Can you work these out from the model? Positions are in its coordinate system, mm. A direction names the side the tool comes from. Coordinates: 2 decimals unless noted, no trailing zeros. Order: outer loops, then holes, each group sorted by start corner. A loop starts at its lowest first (then second) coordinate and runs counter-clockwise, first axis right, second up. Notation, with made-up numbers: (0, -33) -> (58, -33) arc R16 cw to (58, -27) -> close; hole circle Ø2 at (-40, 73.25). An arc over 180 degrees is marked (long way). Write item = value, one per line. Start each with the question number.
from build123d import *

# Parameters (mm, degrees)
GRIPPER_ATTACHMENT_BASE_SKETCH_W   = 12
GRIPPER_ATTACHMENT_BASE_SKETCH_H   = 15
GRIPPER_ATTACHMENT_BASE_DEPTH      = 35.0588586
THICKENER_BASE_DEPTH               = 6
THICKNESS_CUTOFF_SKETCH_W          = 51.475312709
THICKNESS_CUTOFF_SKETCH_H          = 66.937611181
THICKNESS_CUTOFF_DEPTH             = 63.622352222
EXCESS_MATERIAL_CUTOFF_DEPTH       = 530.479784495
EXCESS_MATERIAL_CUTOFF_DEPTH_BACK  = 530.479784495
FINGER_CAVITY_CUTOUT_SKETCH_W      = 6.5
FINGER_CAVITY_CUTOUT_SKETCH_H      = 22
FINGER_CAVITY_CUTOUT_DEPTH         = 15
SCREW_THROUGH_HOLES_SKETCH_R       = 2.25
SCREW_THROUGH_HOLES_DEPTH          = 63.800756824
SOCKET_RECESSES_SKETCH_R           = 3.75
SOCKET_RECESSES_DEPTH              = 2.3625
SHAPING_TO_ELECTRONICS_PLATE_DEPTH = 35.058859


with BuildPart() as part:
    # Gripper Attachment Base Sketch → Gripper Attachment Base (new body)
    with BuildSketch(Plane.XY):
        Rectangle(GRIPPER_ATTACHMENT_BASE_SKETCH_W, GRIPPER_ATTACHMENT_BASE_SKETCH_H)
    extrude(amount=GRIPPER_ATTACHMENT_BASE_DEPTH)

    # Thickener Base Sketch → Thickener Base (add)
    with BuildSketch(Plane(origin=(6, 0, 0), x_dir=(0, 0, -1), z_dir=(1, 0, 0))):
        with BuildLine():
            Line((0, 7.5), (-35.0588586, 7.5))
            Line((-35.0588586, 7.5), (-35.0588586, -48.8959251))
            ThreePointArc((-35.0588586, -48.8959251), (-17.5294293, -38.525001297), (0, -48.8959251))
            Line((0, -48.8959251), (0, 7.5))
        make_face()
    extrude(amount=THICKENER_BASE_DEPTH)

    # Thickness Cutoff Sketch → Thickness Cutoff (cut, through all)
    with BuildSketch(Plane(origin=(12.174072963, -0.29408868, 0), x_dir=(0, 0, -1), z_dir=(0.9997083481115524, -0.02414992165766464, 0))):
        with Locations((-17.603923241, -21.483184787)):
            Rectangle(THICKNESS_CUTOFF_SKETCH_W, THICKNESS_CUTOFF_SKETCH_H)
    extrude(amount=THICKNESS_CUTOFF_DEPTH, mode=Mode.SUBTRACT)

    # Excess Material Cutoff Sketch → Excess Material Cutoff (cut, two sides: drawn at the far end of the back side and taken through both)
    with BuildSketch(Plane(origin=(0, -520.681520523, 0), x_dir=(0, 0, 1), z_dir=(1, 0, 0)).offset(-EXCESS_MATERIAL_CUTOFF_DEPTH_BACK)):
        Polygon((7.0294293, -528.181520523), (0, -528.181520523), (0, -513.181520523), (7.0294293, -524.181520523), align=None)
        Polygon((28.0294293, -528.181520523), (35.0588586, -528.181520523), (35.0588586, -513.181520523), (28.0294293, -524.181520523), align=None)
    extrude(amount=EXCESS_MATERIAL_CUTOFF_DEPTH + EXCESS_MATERIAL_CUTOFF_DEPTH_BACK, mode=Mode.SUBTRACT)

    # Finger Cavity Cutout Sketch → Finger Cavity Cutout (cut)
    with BuildSketch(Plane(origin=(0, 7.5, 0), x_dir=(1, 0, 0), z_dir=(0, 1, 0))):
        with Locations((1.6125, -17.5294293)):
            Rectangle(FINGER_CAVITY_CUTOUT_SKETCH_W, FINGER_CAVITY_CUTOUT_SKETCH_H)
    extrude(amount=-FINGER_CAVITY_CUTOUT_DEPTH, mode=Mode.SUBTRACT)

    # Screw Through-Holes Sketch → Screw Through-Holes (cut, through all)
    with BuildSketch(Plane.ZY.offset(6)):
        with Locations(Location((11.5294293, -0.5, 0), (0, 0, 270))):
            Circle(SCREW_THROUGH_HOLES_SKETCH_R)
        with Locations(Location((23.5294293, -0.5, 0), (0, 0, 270))):
            Circle(SCREW_THROUGH_HOLES_SKETCH_R)
    extrude(amount=-SCREW_THROUGH_HOLES_DEPTH, mode=Mode.SUBTRACT)

    # Socket Recesses Sketch → Socket Recesses (cut)
    with BuildSketch(Plane.ZY.offset(6)):
        with Locations(Location((11.5294293, -0.5, 0), (0, 0, 270))):
            Circle(SOCKET_RECESSES_SKETCH_R)
        with Locations(Location((23.5294293, -0.5, 0), (0, 0, 270))):
            Circle(SOCKET_RECESSES_SKETCH_R)
    extrude(amount=-SOCKET_RECESSES_DEPTH, mode=Mode.SUBTRACT)

    # Shaping to Electronics Plate Sketch → Shaping to Electronics Plate (add, through all)
    with BuildSketch(Plane.XY):
        Polygon((-6, -7.5), (-3, -11.2), (-3, -7.5), align=None)
    extrude(amount=SHAPING_TO_ELECTRONICS_PLATE_DEPTH)


solid = part.part
(1) Imagine slicing it at D-D (z = 32.5). Write out the boundary of the cut face in (x, y).
(2) Thinking about a two-plate mould opening in Z: for faces 4 (the face through (-3.638, 0, 9)), 5 (the face through (2.874, -2.077, 3.466)), 6 (the face through (-4, -9, 35.059)), which applies, +Z half, -Z half, draft (parallel to the pull), parting line (faces both ways), or undercut?
(3) Imagine slicing it at C-C (z = 22.5). Write out the boundary of the cut face in (x, y), plus the area to 3 significant figures.
(4) Imagine slicing it at A-A (x = 2). Write out the boundary of the cut face in (y, z), plus the area to 3 significant figures.
(5) If I drill on L1, parallel to Z at x = -2.4, y = -0.5; L2, parallel to X at y = -6, z = 14.5; L3, parallel to Z at x = -5, y = -3, over which ranges is the centre line in solid material (lowest first)? Write a range as from..to.
(6) For faces 1 (the face through (8, 5, 28.029)), 2 (the face through (-3.638, 0, 21)), 3 (the face through (-1.638, 0, 18)), which set-ups out of +Z, -Z, +X, -X, +Y, -Y let a thin tool reach every point of the face, with its end or its side?
(7) For P1, Ø17.5, axis at y = -20.5, z = 20, coming from the -X side; P2, Ø10, axis at x = 4, z = 18.5, coming from the -Y side; P3, Ø7, axis at x = 2, y = -1.5, coming from the -Z side, each with a flat end and sliding along its axis, tell me the tip position at first contact or that it passes through.
(8) Imagine slicing it at B-B (y = -0.5). Count the separate pieces of the cut face and the enclosed holes in it, plus the area to 3 significant figures.
Result set:
q1.outline = (-6, -7.5) -> (-3, -11.2) -> (-3, -7.5) -> (6, -7.5) -> (6, -45.26) -> (11.09, -45.26) -> (12, -7.5) -> (12, -3.5) -> (-6, -3.5) -> close
q2.face_4 = undercut
q2.face_5 = -Z half
q2.face_6 = +Z half
q3.outline = (-6, -7.5) -> (-3, -11.2) -> (-3, -7.5) -> (-1.64, -7.5) -> (-1.64, -2.5) -> (-3.64, -2.5) -> (-3.64, -4.11) -> (-6, -4.11) -> close; (-6, 3.11) -> (-3.64, 3.11) -> (-3.64, 1.5) -> (-1.64, 1.5) -> (-1.64, 7.5) -> (-6, 7.5) -> close; (4.86, -7.5) -> (6, -7.5) -> (6, -39.15) -> (11.24, -39.15) -> (12, -7.5) -> (12, -2.5) -> (4.86, -2.5) -> close; (4.86, 1.5) -> (12, 1.5) -> (12, 7.5) -> (4.86, 7.5) -> close
q3.area = 302 mm2
q4.outline = (-7.5, 0) -> (2.72, 6.53) -> (-7.5, 6.53) -> close; (-7.5, 28.53) -> (2.72, 28.53) -> (-7.5, 35.06) -> close
q4.area = 66.7 mm2
q5.L1 = 4.47..9.28, 13.78..21.28, 25.78..30.59
q5.L2 = -6..-1.64, 4.86..12
q5.L3 = 2.88..8.73, 14.32..20.73, 26.32..32.18
q6.face_1 = +Z, +X, -X, +Y
q6.face_2 = -X
q6.face_3 = +Y, -Y
q7.P1 = 6
q7.P2 = -39.31
q7.P3 = 1.6
q8.separate_pieces = 4
q8.enclosed_holes = 0
q8.area = 209 mm2
